```python
from build123d import *

# Parameters (mm, degrees)
SKETCH1_R           = 5
SKETCH1_R_2         = 1.5
BOSS_EXTRUDE2_DEPTH = 26
SKETCH2_R           = 6.25
BOSS_EXTRUDE3_DEPTH = 2
CUT_EXTRUDE1_START  = -2
SKETCH3_R           = 5
CUT_EXTRUDE1_DEPTH  = 2
SKETCH5_R           = 12.5
BOSS_EXTRUDE4_DEPTH = 30


with BuildPart() as part:
    # Sketch1 → Boss-Extrude2 (new body)
    with BuildSketch(Plane(origin=(0, 0, 0), x_dir=(1, 0, 0), z_dir=(0, 1, 0))):
        with BuildLine():
            Line((-19.568980619, 0), (53.439105934, 9.332584612))
            ThreePointArc((53.439105934, 9.332584612), (71.14040073, -6.25), (53.439105934, -21.832584612))
            Line((53.439105934, -21.832584612), (-19.568980619, -12.5))
            ThreePointArc((-19.568980619, -12.5), (-25.818980619, -6.25), (-19.568980619, 0))
        make_face()
        with Locations(Location((-19.568980619, -6.25, 0), (0, 0, 90))):
            Circle(SKETCH1_R, mode=Mode.SUBTRACT)
        with Locations(Location((22.660710056, -6.25, 0), (0, 0, 90))):
            Circle(SKETCH1_R_2, mode=Mode.SUBTRACT)
    extrude(amount=BOSS_EXTRUDE2_DEPTH)

    # Sketch2 → Boss-Extrude3 (add)
    with BuildSketch(Plane(origin=(0, 26, 0), x_dir=(1, 0, 0), z_dir=(0, 1, 0))):
        with Locations(Location((-19.568980619, -6.25, 0), (0, 0, 270))):
            Circle(SKETCH2_R)
    extrude(amount=BOSS_EXTRUDE3_DEPTH)

    # Sketch3 → Cut-Extrude1 (cut)
    with BuildSketch(Plane(origin=(0, 28, 0), x_dir=(1, 0, 0), z_dir=(0, 1, 0)).offset(CUT_EXTRUDE1_START)):
        with Locations(Location((-19.568980619, -6.25, 0), (0, 0, 90))):
            Circle(SKETCH3_R)
    extrude(amount=CUT_EXTRUDE1_DEPTH, mode=Mode.SUBTRACT)

    # Sketch5 → Boss-Extrude4 (add)
    with BuildSketch(Plane(origin=(0, 26, 0), x_dir=(1, 0, 0), z_dir=(0, 1, 0))):
        with Locations(Location((54.591675649, -6.337344707, 0), (0, 0, 90))):
            Circle(SKETCH5_R)
    extrude(amount=BOSS_EXTRUDE4_DEPTH)


solid = part.part
```
Geometry check sheet. Reference: the model listing, model coordinates, mm. A direction names the side the tool comes from. Coordinates: 2 decimals unless noted, no trailing zeros. Order: outer loops, then holes, each group sorted by start corner. A loop starts at its lowest first (then second) coordinate and runs counter-clockwise, first axis right, second up. Notation, with made-up numbers: (25.25, 2) - (42.25, 2) arc R26 ccw to (42.25, 25) - close; hole circle Ø9 at (-8.5, 24). An arc over 180 degrees is marked (long way). Use one line per item in the form item = value.
1. Section check B-B (x = 64). Record the boundary of the cut face in (y, z).
Here are the results:
outline = (0, -6.92) - (26, -6.92) - (26, -1.89) - (56, -1.89) - (56, 14.57) - (26, 14.57) - (26, 19.42) - (0, 19.42) - close
2. Gauge pin test, flat ends, axial feed: pin 1 (2 mm diameter, centred on y = 19.5, z = -2, fed in from +X); pin 2 (10 mm diameter, centred on y = 39.5, z = 15, fed in from +X); pin 3 (3 mm diameter, centred on x = 37.5, z = 4.5, fed in from +Y). Record the tip position at first contact, or that the pin passes through.
Here are the results:
pin_1 = 69.37
pin_2 = 66.54
pin_3 = 26
3. Access from +Z, -Z, +X, -X, +Y, -Y to the whole of each face (thin tool, end or side, straight path). Record for faces 5 (the face through (-25.114, 13.804, 9.134)), 6 (the face through (17.446, 12.818, 17.232)).
Here are the results:
face_5 = +Y
face_6 = +Z, -X, +Y, -Y
4. Section check A-A (z = 6.25). Record the boundary of the cut face in (x, y).
Here are the results:
outline = (-25.82, 0) - (-24.57, 0) - (-24.57, 28) - (-25.82, 28) - close; (-14.57, 0) - (21.16, 0) - (21.16, 26) - (-13.32, 26) - (-13.32, 28) - (-14.57, 28) - close; (24.16, 0) - (71.14, 0) - (71.14, 26) - (67.09, 26) - (67.09, 56) - (42.09, 56) - (42.09, 26) - (24.16, 26) - close
5. Section check D-D (y = 47). Record the boundary of the cut face in (x, z), then the cut area to 3 significant figures.
Here are the results:
outline = circle Ø25 at (54.59, 6.34)
area = 491 mm²
6. Scan lines: line 1 (X direction, y = 13.75, z = 6.25); line 2 (Y direction, x = 13.5, z = 1); line 3 (Z direction, x = 60, y = 46). Record each from-to range of solid material in increasing order.
Here are the results:
line_1 = -25.82 to -24.57, -14.57 to 21.16, 24.16 to 71.14
line_2 = 0 to 26
line_3 = -4.93 to 17.61
7. Section check C-C (z = -2.5). Record the boundary of the cut face in (x, y), then the cut area to 3 significant figures.
Here are the results:
outline = (-0.01, 0) - (68.48, 0) - (68.48, 26) - (63.43, 26) - (63.43, 56) - (45.75, 56) - (45.75, 26) - (-0.01, 26) - close
area = 2,310 mm²
8. Draft check along Z on faces 1 (the face through (-15, 28, 3)), 2 (the face through (-21.07, 13.8, 1.48)), 3 (the face through (21.65, 12.82, 7.36)), 4 (the face through (65.68, 40.79, 0.57)). Enter one of: pulls with the +Z half, pulls with the -Z half, needs draft (parallel to the pull), parting line crosses it, or undercut.
Here are the results:
face_1 = needs draft
face_2 = undercut
face_3 = undercut
face_4 = parting line crosses it
